from build123d import *

# Parameters (mm, degrees)
SKETCH1_W           = 200.025
SKETCH1_H           = 260.35
BOSS_EXTRUDE1_DEPTH = 3.175
SKETCH8_R           = 1.55
SKETCH8_R_2         = 1.0499979
CUT_EXTRUDE7_DEPTH  = 4.175
SKETCH9_W           = 50.8
SKETCH9_H           = 127
CUT_EXTRUDE8_DEPTH  = 4.175
FILLET1_R           = 12.7
CUT_EXTRUDE9_DEPTH  = 4.175
SKETCH15_W          = 6.35
SKETCH15_H          = 15.24
CUT_EXTRUDE12_DEPTH = 4.175
SKETCH16_R          = 1.5
SKETCH16_R_2        = 9
CUT_EXTRUDE13_DEPTH = 4.175


with BuildPart() as part:
    # Sketch1 → Boss-Extrude1 (new body)
    with BuildSketch(Plane(origin=(0, 0, 0), x_dir=(0, 0, -1), z_dir=(1, 0, 0))):
        Rectangle(SKETCH1_W, SKETCH1_H)
    extrude(amount=BOSS_EXTRUDE1_DEPTH)

    # Sketch8 → Cut-Extrude7 (cut, through all)
    with BuildSketch(Plane.ZY):
        with Locations((87.3125, 9.525)):
            Circle(SKETCH8_R)
        with Locations((-72.3175, 18.9250066)):
            Circle(SKETCH8_R_2)
        with Locations((-72.3175, 12.4249942)):
            Circle(SKETCH8_R_2)
    extrude(amount=-CUT_EXTRUDE7_DEPTH, mode=Mode.SUBTRACT)

    # Sketch9 → Cut-Extrude8 (cut, through all)
    with BuildSketch(Plane.ZY):
        with Locations((74.6125, -66.675)):
            Rectangle(SKETCH9_W, SKETCH9_H)
    extrude(amount=-CUT_EXTRUDE8_DEPTH, mode=Mode.SUBTRACT)

    # Fillet1
    fillet1_edges = [part.edges().sort_by_distance(p)[0] for p in [
        (1.5875, -3.175, 49.2125),
    ]]
    fillet(fillet1_edges, radius=FILLET1_R)

    # Sketch10 → Cut-Extrude9 (cut, through all)
    with BuildSketch(Plane.ZY):
        with BuildLine():
            ThreePointArc((-34.631218673, 67.095364965), (-44.09213985, 39.8142402), (-47.528128749, 11.144346963))
            ThreePointArc((-47.528128749, 11.144346963), (-42.823162504, 6.325000001), (-38.003815542, 11.029966247))
            ThreePointArc((-38.003815542, 11.029966247), (-34.810523806, 37.674794334), (-26.017864022, 63.028948034))
            ThreePointArc((-26.017864022, 63.028948034), (-28.291332832, 69.36883393), (-34.631218673, 67.095364965))
        make_face()
    extrude(amount=-CUT_EXTRUDE9_DEPTH, mode=Mode.SUBTRACT)

    # Sketch15 → Cut-Extrude12 (cut, through all)
    with BuildSketch(Plane(origin=(3.175, 0, 0), x_dir=(0, 0, -1), z_dir=(1, 0, 0))):
        with Locations((77.4925, -1.5450058)):
            Rectangle(SKETCH15_W, SKETCH15_H)
        with Locations((77.4925, -42.1850058)):
            Rectangle(SKETCH15_W, SKETCH15_H)
    extrude(amount=-CUT_EXTRUDE12_DEPTH, mode=Mode.SUBTRACT)

    # Sketch16 → Cut-Extrude13 (cut, through all)
    with BuildSketch(Plane(origin=(3.175, 0, 0), x_dir=(0, 0, -1), z_dir=(1, 0, 0))):
        with Locations((82.075, -125.4125)):
            Circle(SKETCH16_R)
        with Locations((82.075, -76.4125)):
            Circle(SKETCH16_R)
        with Locations((92.075, -125.4125)):
            Circle(SKETCH16_R)
        with Locations((92.075, -76.4125)):
            Circle(SKETCH16_R)
        with Locations((87.075, -110.5624916)):
            Circle(SKETCH16_R_2)
    extrude(amount=-CUT_EXTRUDE13_DEPTH, mode=Mode.SUBTRACT)


solid = part.part
Could you check a few things on this model? Use its own coordinates, in mm. A direction names the side the tool comes from. Give positions to 0.01 mm unless a question says otherwise; leave off trailing zeros. Order: outer loops, then holes, each group sorted by start corner. A loop starts at its lowest first (then second) coordinate and runs counter-clockwise, first axis right, second up. Notation, with made-up numbers: (72, 45.25) -> (97, 45.25) arc R24 cw to (97, 74.25) -> close; hole circle Ø1 at (18.25, 71). An arc over 180 degrees is marked (long way). Return JSON: item names as keys, results as strings.
1. Imagine slicing it at A-A on y = 54. List the corners of the cut face in (x, z) for me (1 decimal).
Answer list:
{"outline": "(0, -100) -> (3.2, -100) -> (3.2, -40) -> (0, -40) -> close; (0, -29.9) -> (3.2, -29.9) -> (3.2, 100) -> (0, 100) -> close"}
2. For pin 1 Ø11 at (y, z) = (-110.56, -87.08) entering from +X; pin 2 Ø1.6 at (x, y) = (1, -44) entering from +Z; pin 3 Ø1.5 at (x, z) = (1, 71.5) entering from -Y (3 decimals), each with a flat end and sliding along its axis, tell me the tip position at first contact or that it passes through.
Answer list:
{"pin 1": "passes through", "pin 2": "stops at z = 49.21", "pin 3": "stops at y = -3.175"}
3. Imagine slicing it at B-B on x = 1.6. Give the number of separate pieces and of enclosed holes in the cut face, then the cut area to 3 significant figures.
Answer list:
{"separate pieces": "1", "enclosed holes": "11", "area": "44,600 mm2"}
4. Imagine slicing it at D-D on y = -113.5. List the corners of the cut face in (x, z) for me (1 decimal).
Answer list:
{"outline": "(0, -100) -> (3.2, -100) -> (3.2, -95.6) -> (0, -95.6) -> close; (0, -78.6) -> (3.2, -78.6) -> (3.2, 49.2) -> (0, 49.2) -> close"}
5. Imagine slicing it at C-C on z = 65. List the corners of the cut face in (x, y) for me (3 decimals).
Answer list:
{"outline": "(0, -3.175) -> (3.175, -3.175) -> (3.175, 130.175) -> (0, 130.175) -> close"}
6. On a 3-axis mill with a long thin cutter (end or side, diameter ignored), from which of +Z, -Z, +X, -X, +Y, -Y can I reach the whole of each face in a straight line? I mean faces 4 (the cylindrical face through (1.565, 37.308, -34.895)), 5 (the flat face through (3.175, 2, 1)). Say none if no direction works.
Answer list:
{"face 4": "+X, -X", "face 5": "+Z, -Z, +X, +Y, -Y"}
7. Thinking about a two-plate mould opening in Y: for faces 1 (the flat face through (0, 2, 1)), 2 (the cylindrical face through (1.565, 69.323, -28.197)), 3 (the cylindrical face through (1.61, -6.8, 53.03)), which applies, pulls with the +Y half, pulls with the -Y half, needs draft (parallel to the pull), parting line crosses it, or undercut?
Answer list:
{"face 1": "needs draft", "face 2": "undercut", "face 3": "pulls with the -Y half"}
8. I need wall thicknesses on line 1 (Y direction, x = 0.7, z = -75.5) (3 decimals); line 2 (Y direction, x = 1.65, z = -79.5) (3 decimals); line 3 (Z direction, x = 2.85, y = 3). Which ranges of each line are inside material? Lowest first, please. Write a range as from..to.
Answer list:
{"line 1": "y = -130.175..-49.805, -34.565..-9.165, 6.075..130.175", "line 2": "y = -130.175..-115.422, -105.703..-49.805, -34.565..-9.165, 6.075..130.175", "line 3": "z = -100.01..-80.67, -74.32..100.01"}
